Model file for the job. Use its own axes, mm. A direction names the side the tool comes from. Round coordinates to 2 decimals unless told otherwise and drop trailing zeros. Order: outer loops, then holes, each group sorted by start corner. A loop starts at its lowest first (then second) coordinate and runs counter-clockwise, first axis right, second up. Notation, with made-up numbers: (39, 19.5) - (94, 19.5) arc R27 ccw to (94, 52.5) - close; hole circle Ø6 at (-7, 37.25). An arc over 180 degrees is marked (long way). Answer as CSV lines item,"result". Start each with the question number.
1. 3-axis set-ups, long thin cutter, end or side, ignore diameter. For faces 1 (the face through (0, 3, -17.5)), 2 (the face through (-42.53, 4.02, -20.29)), 3 (the face through (-34.5, 3, 20)): which of +Z, -Z, +X, -X, +Y, -Y reach the whole face in a straight line?
2. Band-saw the part on B-B on y = 1.55. List the corners of the cut face in (x, z).
3. Band-saw the part on A-A on x = -40.5. List the corners of the cut face in (y, z), then the cut area to 4 significant figures.
4. Band-saw the part on C-C on x = -7. List the corners of the cut face in (y, z).
5. Wall check: line 1 along Z through (x, y) = (40.5, 1.45); line 2 along X through (y, z) = (4.75, 22.5); line 3 along X through (y, z) = (0.6, -22.5). Give the ranges that are in metal, low to high. Write a range as [from, to].
6. Pin check, flat tips, straight feed: pin 1 Ø5 at (x, z) = (40.5, 22.5) entering from +Y; pin 2 Ø2 at (x, y) = (-34, 4.5) entering from -Z; pin 3 Ø5 at (x, z) = (-41.5, -22.5) entering from +Y; pin 4 Ø1.5 at (x, y) = (9, 4) entering from +Z. Stop position of each tip, or through.
7. Pull direction Z, two halves, no side cores. Call faces 4 (the face through (0, 3, 17.5)), 5 (the face through (42, 2.5, 21)), 6 (the face through (-40.6, 2.7, -28.5)): released by +Z, released by -Z, zero draft, split by the parting line, or undercut.
```python
from build123d import *

# Parameters (mm, degrees)
SKETCH_1_R          = 1.5
SKETCH_1_W          = 69
SKETCH_1_H          = 10
EXTRUDE_3_DEPTH     = 5.5
SKETCH_2_R          = 3
CUT_EXTRUDE_1_DEPTH = 3


with BuildPart() as part:
    # 草图1 → 凸台-拉伸3 (new body)
    with BuildSketch(Plane(origin=(0, 0, 0), x_dir=(1, 0, 0), z_dir=(0, 1, 0))):
        with BuildLine():
            Line((46.5, 22.5), (46.5, -22.5))
            ThreePointArc((46.5, -22.5), (40.5, -28.5), (34.5, -22.5))
            Line((34.5, -22.5), (34.5, -17.5))
            Line((34.5, -17.5), (-34.5, -17.5))
            Line((-34.5, -17.5), (-34.5, -22.5))
            ThreePointArc((-34.5, -22.5), (-40.5, -28.5), (-46.5, -22.5))
            Line((-46.5, -22.5), (-46.5, 22.5))
            ThreePointArc((-46.5, 22.5), (-40.5, 28.5), (-34.5, 22.5))
            Line((-34.5, 22.5), (-34.5, 17.5))
            Line((-34.5, 17.5), (34.5, 17.5))
            Line((34.5, 17.5), (34.5, 22.5))
            ThreePointArc((34.5, 22.5), (40.5, 28.5), (46.5, 22.5))
        make_face()
        with Locations(Location((40.5, 22.5, 0), (0, 0, 270))):
            Circle(SKETCH_1_R, mode=Mode.SUBTRACT)
        with Locations(Location((40.5, -22.5, 0), (0, 0, 90))):
            Circle(SKETCH_1_R, mode=Mode.SUBTRACT)
        with Locations(Location((-40.5, -22.5, 0), (0, 0, 270))):
            Circle(SKETCH_1_R, mode=Mode.SUBTRACT)
        with Locations(Location((-40.5, 22.5, 0), (0, 0, 90))):
            Circle(SKETCH_1_R, mode=Mode.SUBTRACT)
        Rectangle(SKETCH_1_W, SKETCH_1_H, mode=Mode.SUBTRACT)
    extrude(amount=EXTRUDE_3_DEPTH)

    # 草图2 → 切除-拉伸1 (cut)
    with BuildSketch(Plane(origin=(0, 5.5, 0), x_dir=(1, 0, 0), z_dir=(0, 1, 0))):
        with Locations(Location((40.5, 22.5, 0), (0, 0, 270))):
            Circle(SKETCH_2_R)
        with Locations(Location((40.5, -22.5, 0), (0, 0, 90))):
            Circle(SKETCH_2_R)
        with Locations(Location((-40.5, -22.5, 0), (0, 0, 270))):
            Circle(SKETCH_2_R)
        with Locations(Location((-40.5, 22.5, 0), (0, 0, 90))):
            Circle(SKETCH_2_R)
    extrude(amount=-CUT_EXTRUDE_1_DEPTH, mode=Mode.SUBTRACT)


solid = part.part
```
Reply:
1,face 1,"-Z, +Y, -Y"
1,face 2,"+Y"
1,face 3,"+Z, +Y, -Y"
2,outline,"(-46.5, -22.5) arc R6 ccw to (-34.5, -22.5) - (-34.5, -17.5) - (34.5, -17.5) - (34.5, -22.5) arc R6 ccw to (46.5, -22.5) - (46.5, 22.5) arc R6 ccw to (34.5, 22.5) - (34.5, 17.5) - (-34.5, 17.5) - (-34.5, 22.5) arc R6 ccw to (-46.5, 22.5) - close; hole circle Ø3 at (-40.5, -22.5); hole circle Ø3 at (-40.5, 22.5); hole (-34.5, -5) - (34.5, -5) - (34.5, 5) - (-34.5, 5) - close; hole circle Ø3 at (40.5, -22.5); hole circle Ø3 at (40.5, 22.5)"
3,outline,"(0, -28.5) - (5.5, -28.5) - (5.5, -25.5) - (2.5, -25.5) - (2.5, -24) - (0, -24) - close; (0, -21) - (2.5, -21) - (2.5, -19.5) - (5.5, -19.5) - (5.5, 19.5) - (2.5, 19.5) - (2.5, 21) - (0, 21) - close; (0, 24) - (2.5, 24) - (2.5, 25.5) - (5.5, 25.5) - (5.5, 28.5) - (0, 28.5) - close"
3,area,"262.5 mm2"
4,outline,"(0, -17.5) - (5.5, -17.5) - (5.5, -5) - (0, -5) - close; (0, 5) - (5.5, 5) - (5.5, 17.5) - (0, 17.5) - close"
5,line 1,"z = [-28.5, -24], [-21, 21], [24, 28.5]"
5,line 2,"x = [-46.5, -43.5], [-37.5, -34.5], [34.5, 37.5], [43.5, 46.5]"
5,line 3,"x = [-46.5, -42], [-39, -34.5], [34.5, 39], [42, 46.5]"
6,pin 1,"stops at y = 2.5"
6,pin 2,"stops at z = -24.9"
6,pin 3,"stops at y = 5.5"
6,pin 4,"stops at z = 17.5"
7,face 4,"released by +Z"
7,face 5,"undercut"
7,face 6,"released by -Z"
